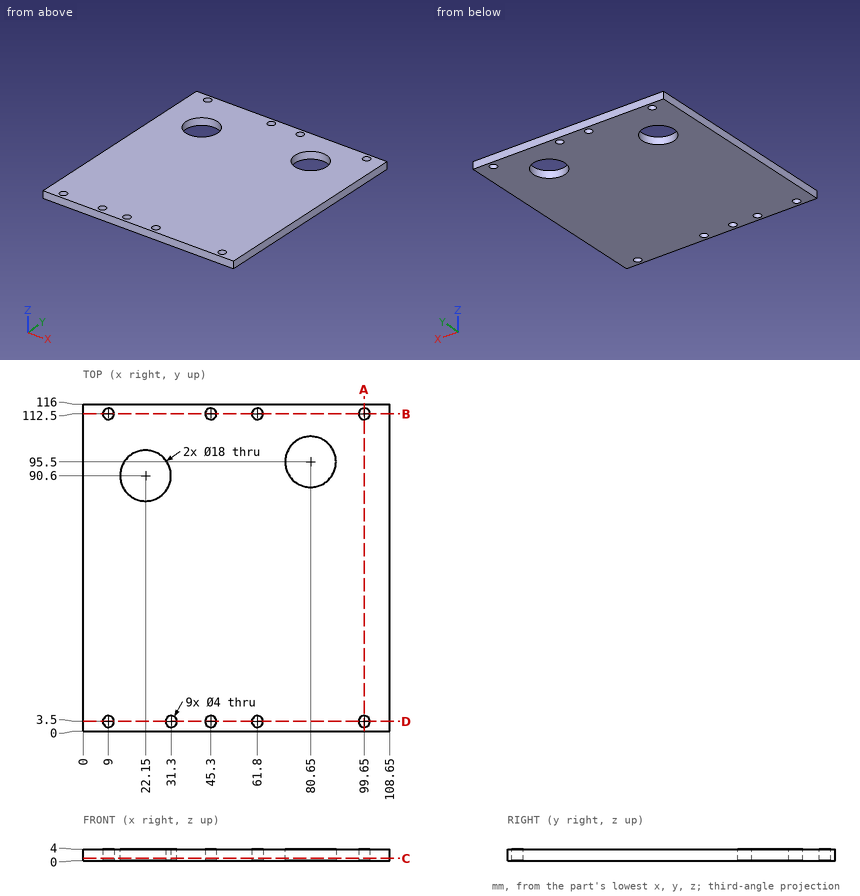
Design review of the part shown in the three views and the two pictorial views. Dimensions are in mm from the part's minimum x, y and z. Round coordinates to 2 decimals unless told otherwise and drop trailing zeros. Order: outer loops, then holes, each group sorted by start corner. A loop starts at its lowest first (then second) coordinate and runs counter-clockwise, first axis right, second up. Notation, with made-up numbers: (-31.5, -1.75) - (-25.5, -1.75) arc R25 cw to (-25.5, 29.25) - close; hole circle Ø4 at (69.25, -19.75). An arc over 180 degrees is marked (long way). Answer in a Markdown table with one row per item.
(1) Take a section at A-A on x = 99.65. Write out the cut boundary in (y, z).
Result set:
| item | result |
|---|---|
| outline | (0, 0) - (1.5, 0) - (1.5, 4) - (0, 4) - close; (5.5, 0) - (110.5, 0) - (110.5, 4) - (5.5, 4) - close; (114.5, 0) - (116, 0) - (116, 4) - (114.5, 4) - close |
(2) For line 1 (Y direction, x = 99.65, z = 1.75); line 2 (X direction, y = 112.5, z = 1.5); line 3 (Y direction, x = 22, z = 0.55), list the stretches that pass through material, from the lowest coordinate up. Write a range as from..to.
Result set:
| item | result |
|---|---|
| line 1 | y = 0..1.5, 5.5..110.5, 114.5..116 |
| line 2 | x = 0..7, 11..43.3, 47.3..59.8, 63.8..97.65, 101.65..108.65 |
| line 3 | y = 0..81.6, 99.6..116 |
(3) Take a section at D-D on y = 3.5. Write out the cut boundary in (x, z), plus the area to 3 significant figures.
Result set:
| item | result |
|---|---|
| outline | (0, 0) - (7, 0) - (7, 4) - (0, 4) - close; (11, 0) - (29.3, 0) - (29.3, 4) - (11, 4) - close; (33.3, 0) - (43.3, 0) - (43.3, 4) - (33.3, 4) - close; (47.3, 0) - (59.8, 0) - (59.8, 4) - (47.3, 4) - close; (63.8, 0) - (97.65, 0) - (97.65, 4) - (63.8, 4) - close; (101.65, 0) - (108.65, 0) - (108.65, 4) - (101.65, 4) - close |
| area | 355 mm2 |
(4) Take a section at B-B on y = 112.5. Write out the cut boundary in (x, z).
Result set:
| item | result |
|---|---|
| outline | (0, 0) - (7, 0) - (7, 4) - (0, 4) - close; (11, 0) - (43.3, 0) - (43.3, 4) - (11, 4) - close; (47.3, 0) - (59.8, 0) - (59.8, 4) - (47.3, 4) - close; (63.8, 0) - (97.65, 0) - (97.65, 4) - (63.8, 4) - close; (101.65, 0) - (108.65, 0) - (108.65, 4) - (101.65, 4) - close |
(5) Take a section at C-C on z = 0.85. Count the separate pieces of the cut face and the enclosed holes in it, plus the area to 3 significant figures.
Result set:
| item | result |
|---|---|
| separate pieces | 1 |
| enclosed holes | 11 |
| area | 12,000 mm2 |
